The model under review builds one solid part; all positions refer to its coordinate system, in mm. Face numbers are marked on the shaded views. A direction names the side the tool comes from. Round coordinates to 2 decimals unless told otherwise and drop trailing zeros. Order: outer loops, then holes, each group sorted by start corner. A loop starts at its lowest first (then second) coordinate and runs counter-clockwise, first axis right, second up.
1) Consider section C-C (z = 3.25). Give the boundary of the cut face in (x, y).
2) Clearance check with flat-ended pins moving along their axes: P1, Ø2, axis at x = 4.5, z = -3, coming from the +Y side; P2, Ø0.9, axis at y = 0.5, z = 0.5, coming from the -X side; P3, Ø1.5, axis at x = -0.5, z = 0, coming from the +Y side; P4, Ø6, axis at x = 4.5, y = -9.5, coming from the -Z side. State where each tip first meets the part, or that it passes through.
3) Consider section D-D (y = -3.5). Give the boundary of the cut face in (x, z).
4) Machinability: for the marked faces 1, 2 and 3, which of the approach directions +Z, -Z, +X, -X, +Y, -Y give a long, thin tool a straight path to every point of the face, cutting with its end or side? Answer none if there is none.
5) Mouldability with a two-part tool opening along Y and no side actions: class the marked faces 4, 5 and 6 as pulls with the +Y half, pulls with the -Y half, needs draft (parallel to the pull), parting line crosses it, or undercut.
6) To check wall thickness, follow L1, parallel to Y at x = -3.25, z = 2.25; L2, parallel to X at y = -15.7, z = 0; L3, parallel to Y at x = 5.25, z = 3. State the ranges of each line that lie inside material, in increasing order.
7) Consider section B-B (y = -18.5). Give the boundary of the cut face in (x, z), then the cut area to 3 significant figures.
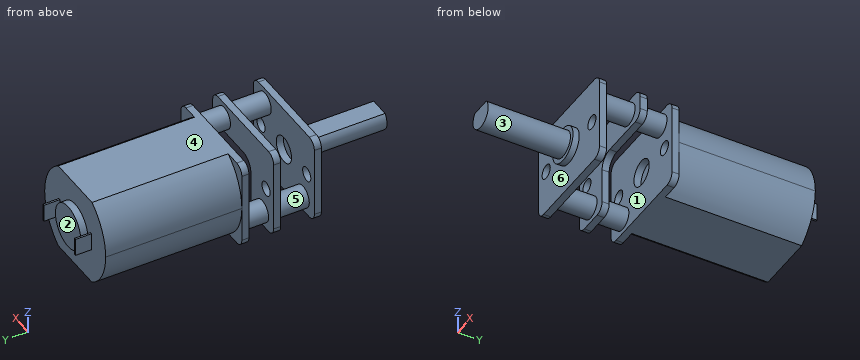
from build123d import *

# Parameters (mm, degrees)
F1_DEPTH      = 15.4
F3_DEPTH      = 0.8
F4_DEPTH      = 1.8
F5_R          = 0.8
F5_R_2        = 1.5
F6_DEPTH      = 9
F7_W          = 3.8
F7_H          = 10
F7_W_2        = 2.8
F8_DEPTH      = 25
F8_DEPTH_BACK = 25
F10_DEPTH     = 1
F12_R         = 1.25
F13_DEPTH     = 7.4
F15_R         = 2
F16_DEPTH     = 0.7
F17_DEPTH     = 1
F18_DEPTH     = 10


with BuildPart() as f1:
    # F0 (on Front) → F1 (new body)
    with BuildSketch(Plane.XZ):
        with BuildLine():
            ThreePointArc((3.3166247904, -5), (5.2867640737, -2.8372743309), (6, 0))
            ThreePointArc((6, 0), (5.2867640737, 2.8372743309), (3.3166247904, 5))
            Line((3.3166247904, 5), (-3.3166247904, 5))
            ThreePointArc((-3.3166247904, 5), (-5.2867640737, 2.8372743309), (-6, 0))
            ThreePointArc((-6, 0), (-5.2867640737, -2.8372743309), (-3.3166247904, -5))
            Line((-3.3166247904, -5), (3.3166247904, -5))
        make_face()
    extrude(amount=F1_DEPTH)

    # F2 (on Front) → F3 (join)
    with BuildSketch(Plane.XZ):
        with BuildLine():
            Line((2.5, 0), (-2.5, 0))
            ThreePointArc((-2.5, 0), (0, -2.5), (2.5, 0))
        make_face()
        with BuildLine():
            ThreePointArc((2.5, 0), (0, 2.5), (-2.5, 0))
            Line((-2.5, 0), (2.5, 0))
        make_face()
    extrude(amount=-F3_DEPTH)

    # F2 (on Front) → F4 (join)
    with BuildSketch(Plane.XZ):
        Polygon((3, 1), (3, 0), (3, -1), (3.2, -1), (3.2, 1), align=None)
        Polygon((-3, 1), (-3.2, 1), (-3.2, -1), (-3, -1), (-3, 0), align=None)
    extrude(amount=-F4_DEPTH)

    # F5 (on face) → F6 (join)
    with BuildSketch(Plane.XZ.offset(15.4)):
        with BuildLine():
            Line((5, 5), (-5, 5))
            ThreePointArc((-5, 5), (-5.7071067812, 4.7071067812), (-6, 4))
            Line((-6, 4), (-6, -4))
            ThreePointArc((-6, -4), (-5.7071067812, -4.7071067812), (-5, -5))
            Line((-5, -5), (5, -5))
            ThreePointArc((5, -5), (5.7071067812, -4.7071067812), (6, -4))
            Line((6, -4), (6, 4))
            ThreePointArc((6, 4), (5.7071067812, 4.7071067812), (5, 5))
        make_face()
        with Locations((-4.5, 0)):
            Circle(F5_R, mode=Mode.SUBTRACT)
        Circle(F5_R_2, mode=Mode.SUBTRACT)
        with Locations((4.5, 0)):
            Circle(F5_R, mode=Mode.SUBTRACT)
    extrude(amount=F6_DEPTH)

    # F7 (on Right) → F8 (cut, two sides)
    with BuildSketch(Plane.YZ) as f8_sk:
        with Locations((-21.7, 0)):
            Rectangle(F7_W, F7_H)
        with Locations((-17.6, 0)):
            Rectangle(F7_W_2, F7_H)
    extrude(amount=-F8_DEPTH, mode=Mode.SUBTRACT)
    extrude(f8_sk.sketch, amount=F8_DEPTH_BACK, mode=Mode.SUBTRACT)

    # F9 (on face) → F10 (cut)
    with BuildSketch(Plane.XZ.offset(19.8)):
        with BuildLine():
            Line((5, 1.5), (0, 1.5))
            ThreePointArc((0, 1.5), (-1.0606601718, 1.0606601718), (-1.5, 0))
            Line((-1.5, 0), (-1.5, -4))
            ThreePointArc((-1.5, -4), (-1.7928932188, -4.7071067812), (-2.5, -5))
            Line((-2.5, -5), (-2.5, -6))
            Line((-2.5, -6), (-1.5, -6))
            Line((-1.5, -6), (7, -6))
            Line((7, -6), (7, 2.5))
            Line((7, 2.5), (6, 2.5))
            ThreePointArc((6, 2.5), (5.7071067812, 1.7928932188), (5, 1.5))
        make_face()
    extrude(amount=-F10_DEPTH, mode=Mode.SUBTRACT)

    # F12 (on offset) → F13 (join)
    with BuildSketch(Plane.XZ.offset(16.2)):
        with Locations((-3.75, -3.25)):
            Circle(F12_R)
        with Locations((3.75, 3.25)):
            Circle(F12_R)
    extrude(amount=F13_DEPTH)

    # F15 (on offset) → F16 (join)
    with BuildSketch(Plane.XZ.offset(24.4)):
        Circle(F15_R)
        with BuildLine():
            ThreePointArc((1.1180339887, 1), (1.4012585384, 0.5352331347), (1.5, 0))
            ThreePointArc((1.5, 0), (-0.5352331347, -1.4012585384), (-1.1180339887, 1))
            ThreePointArc((-1.1180339887, 1), (0, 1.5), (1.1180339887, 1))
        make_face(mode=Mode.SUBTRACT)
    extrude(amount=F16_DEPTH)

    # F15 (on offset) → F17 (join)
    with BuildSketch(Plane.XZ.offset(24.4)):
        with BuildLine():
            Line((-1.1180339887, 1), (1.1180339887, 1))
            ThreePointArc((1.1180339887, 1), (0, 1.5), (-1.1180339887, 1))
        make_face()
        with BuildLine():
            ThreePointArc((-1.1180339887, 1), (-0.5352331347, -1.4012585384), (1.5, 0))
            ThreePointArc((1.5, 0), (1.4012585384, 0.5352331347), (1.1180339887, 1))
            Line((1.1180339887, 1), (-1.1180339887, 1))
        make_face()
    extrude(amount=F17_DEPTH)

    # F15 (on offset) → F18 (join)
    with BuildSketch(Plane.XZ.offset(24.4)):
        with BuildLine():
            ThreePointArc((-1.1180339887, 1), (-0.5352331347, -1.4012585384), (1.5, 0))
            ThreePointArc((1.5, 0), (1.4012585384, 0.5352331347), (1.1180339887, 1))
            Line((1.1180339887, 1), (-1.1180339887, 1))
        make_face()
    extrude(amount=F18_DEPTH)


solid = f1.part
Answer below:
1. outline: (-6, -24.4) - (6, -24.4) - (6, -23.6) - (5, -23.6) - (5, -19.8) - (6, -19.8) - (6, -19) - (5, -19) - (5, -16.2) - (6, -16.2) - (6, -15.4) - (5.04, -15.4) - (5.04, 0) - (-5.04, 0) - (-5.04, -15.4) - (-6, -15.4) - (-6, -16.2) - (2.5, -16.2) - (2.5, -19) - (-6, -19) - (-6, -19.8) - (2.5, -19.8) - (2.5, -23.6) - (-6, -23.6) - close
2. P1: stops at y = 0
2. P2: stops at x = -3.2
2. P3: stops at y = 0.8
2. P4: stops at z = -5
3. outline: (-3.32, -5) - (3.32, -5) arc R6 ccw to (3.32, 5) - (-3.32, 5) arc R6 ccw to start
4. face 1: none
4. face 2: +Z, -Z, +Y
4. face 3: -Y
5. face 4: needs draft
5. face 5: undercut
5. face 6: pulls with the -Y half
6. L1: y = -24.4 to -23.6, -19.8 to -19, -16.2 to 0
6. L2: x = -6 to -5.3, -3.7 to -1.5, 1.5 to 3.7, 5.3 to 6
6. L3: y = -24.4 to -23.6, -19.8 to -19, -16.2 to -15.4
7. outline: circle Ø2.5 at (-3.75, -3.25); circle Ø2.5 at (3.75, 3.25)
7. area: 9.82 mm2
